Geometry check sheet. Reference: the model listing, model coordinates, mm. A direction names the side the tool comes from. Round coordinates to 2 decimals unless told otherwise and drop trailing zeros. Order: outer loops, then holes, each group sorted by start corner. A loop starts at its lowest first (then second) coordinate and runs counter-clockwise, first axis right, second up. Notation, with made-up numbers: M 4,85 L 40,85 A18 cw 40,117 Z; hole C 2,52 d4. An arc over 180 degrees is marked long. Return JSON: item names as keys, results as strings. Group by question number.
```python
from build123d import *

# Parameters (mm, degrees)
EXTRUDE_1_DEPTH     = 41.402
SKETCH_4_R          = 7.112
CUT_EXTRUDE_1_DEPTH = 83.979969858
SKETCH_3_R          = 7.112
CUT_EXTRUDE_2_DEPTH = 83.979969858
SKETCH1_W           = 41.402
SKETCH1_H           = 42.010980282
BOSS_EXTRUDE1_DEPTH = 6.35
SKETCH2_R           = 7.112
CUT_EXTRUDE1_DEPTH  = 80.251737506


with BuildPart() as part:
    # 草图1 → 凸台-拉伸1 (new body)
    with BuildSketch(Plane.XY):
        with BuildLine():
            Line((2.54, 0), (50.8, 0))
            Line((50.8, 0), (50.8, 6.35))
            Line((50.8, 6.35), (8.89, 6.35))
            ThreePointArc((8.89, 6.35), (7.093948776, 7.093948776), (6.35, 8.89))
            Line((6.35, 8.89), (6.35, 50.900980282))
            Line((6.35, 50.900980282), (0, 50.900980282))
            Line((0, 50.900980282), (0, 2.54))
            ThreePointArc((0, 2.54), (0.743948776, 0.743948776), (2.54, 0))
        make_face()
    extrude(amount=EXTRUDE_1_DEPTH)

    # 草图4 → 切除-拉伸1 (cut, through all)
    with BuildSketch(Plane.ZY):
        with Locations((20.701, 28.448)):
            Circle(SKETCH_4_R)
    extrude(amount=-CUT_EXTRUDE_1_DEPTH, mode=Mode.SUBTRACT)

    # 草图3 → 切除-拉伸2 (cut, through all)
    with BuildSketch(Plane(origin=(0, 0, 0), x_dir=(-1, 0, 0), z_dir=(0, -1, 0))):
        with Locations(Location((-31.75, -20.701, 0), (0, 0, 90))):
            Circle(SKETCH_3_R)
    extrude(amount=-CUT_EXTRUDE_2_DEPTH, mode=Mode.SUBTRACT)

    # Sketch1 → Boss-Extrude1 (add)
    with BuildSketch(Plane(origin=(6.35, 0, 0), x_dir=(0, 0, -1), z_dir=(1, 0, 0))):
        with Locations((20.701, 29.895490141)):
            Rectangle(SKETCH1_W, SKETCH1_H)
    extrude(amount=-BOSS_EXTRUDE1_DEPTH)

    # Sketch2 → Cut-Extrude1 (cut, through all)
    with BuildSketch(Plane(origin=(6.35, 0, 0), x_dir=(0, 0, -1), z_dir=(1, 0, 0))):
        with Locations(Location((-20.701, 28.448, 0), (0, 0, 180))):
            Circle(SKETCH2_R)
        with Locations((20.701, 28.448)):
            Circle(SKETCH2_R)
    extrude(amount=-CUT_EXTRUDE1_DEPTH, mode=Mode.SUBTRACT)


solid = part.part
```
Q1. Section check D-D on z = 5.5. Record the cut outline in (x, y).
Q2. Set-up check for faces 5 (the face through (3, 8.89, -20)), 6 (the face through (0.724, 0.764, 20.411)), 7 (the face through (6.35, 30, 1)): record each of +Z, -Z, +X, -X, +Y, -Y from which the full face is reachable in a straight line by a thin tool's end or side.
Q3. Section check C-C on z = 18. Record the cut outline in (x, y), plus the area to 3 significant figures.
Q4. Depth check by flat-ended pin: pin 1 Ø20.5 at (x, z) = (38.5, 12) entering from +Y; pin 2 Ø10 at (x, y) = (12.5, 10) entering from -Z; pin 3 Ø6 at (y, z) = (16, 31.5) entering from +X. Enter the tip coordinate at first touch or a pass-through.
Q5. Section check A-A on x = 31.75. Record the cut outline in (y, z), plus the area to 3 significant figures.
Q6. Section check B-B on y = 25. Record the cut outline in (x, z).
Q7. Release check for a two-part mould opening along Y. For faces 1 (the face through (3.1, 33.3, 15.5)), 2 (the face through (3, 50.901, 1)), 3 (the face through (26, 0, 16)), 4 (the face through (0, 27, 1)) record: +Y half, -Y half, draft (parallel to the pull), parting line (faces both ways), or undercut.
Q8. Material ranges on line 1 along X through (y, z) = (24, -13.5); line 2 along Z through (x, y) = (4, 29.5); line 3 along Z through (x, y) = (31, 5), recorded low to high.
Geometry check:
{
 "1": {"outline": "M 0,2.54 A2.54 ccw 2.54,0 L 50.8,0 L 50.8,6.35 L 8.89,6.35 A2.54 cw 6.35,8.89 L 6.35,50.9 L 0,50.9 Z"},
 "2": {"face 5": "-Z, +X, -X, -Y", "face 6": "+Z, -Z, -X, -Y", "face 7": "+Z, -Z, +X, +Y"},
 "3": {"outline": "M 0,2.54 A2.54 ccw 2.54,0 L 25.17,0 L 25.17,6.35 L 8.89,6.35 A2.54 cw 6.35,8.89 L 6.35,21.87 L 0,21.87 Z; M 0,35.03 L 6.35,35.03 L 6.35,50.9 L 0,50.9 Z; M 38.33,0 L 50.8,0 L 50.8,6.35 L 38.33,6.35 Z", "area": "438 mm^2"},
 "4": {"pin 1": "stops at y = 6.35", "pin 2": "stops at z = 0", "pin 3": "stops at x = 6.35"},
 "5": {"outline": "M 0,0 L 6.35,0 L 6.35,13.59 L 0,13.59 Z; M 0,27.81 L 6.35,27.81 L 6.35,41.4 L 0,41.4 Z", "area": "173 mm^2"},
 "6": {"outline": "M 0,-41.4 L 6.35,-41.4 L 6.35,-26.92 L 0,-26.92 Z; M 0,-14.48 L 6.35,-14.48 L 6.35,14.48 L 0,14.48 Z; M 0,26.92 L 6.35,26.92 L 6.35,41.4 L 0,41.4 Z"},
 "7": {"face 1": "undercut", "face 2": "+Y half", "face 3": "-Y half", "face 4": "draft"},
 "8": {"line 1": "x = 0 to 6.35", "line 2": "z = -41.4 to -27.73, -13.67 to 13.67, 27.73 to 41.4", "line 3": "z = 0 to 13.63, 27.77 to 41.4"}
}
